The listing builds one solid part. Answer for the finished solid, in the listing's coordinates (mm). Face numbers are marked on the shaded views. A direction names the side the tool comes from. Give positions to 0.01 mm unless a question says otherwise; leave off trailing zeros. Loops run counter-clockwise (first coordinate to the right, second up) from the corner with the lowest first, then second, coordinate; pieces in that order, holes last. Notation, with made-up numbers: M -17.75,75 L 24.25,75 A28 cw 24.25,105 Z; hole C -38.5,-31 d9. An arc over 180 degrees is marked long. Return JSON: item names as keys, results as strings.
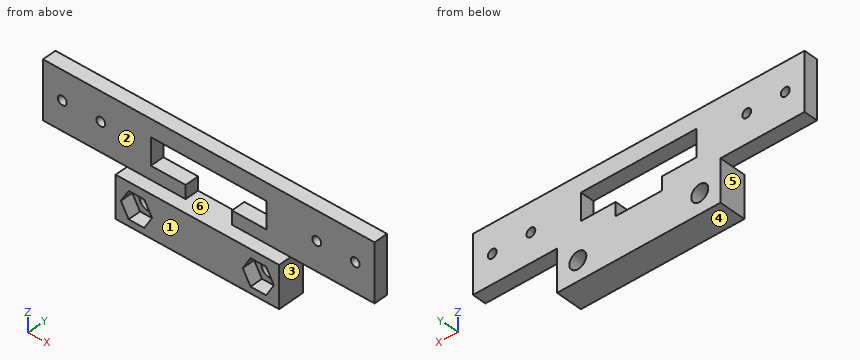
from build123d import *

# Parameters (mm, degrees)
SKETCH1_R           = 1.15
SKETCH1_R_2         = 2.2
BOSS_EXTRUDE2_DEPTH = 3.6
SKETCH2_W           = 42.4
SKETCH2_H           = 10.88
BOSS_EXTRUDE3_DEPTH = 3.3


with BuildPart() as part:
    # Sketch1 → Boss-Extrude2 (new body)
    with BuildSketch(Plane(origin=(0, 0, 0), x_dir=(1, 0, 0), z_dir=(0, 1, 0))):
        Polygon((33, 7.5), (21.2, 7.5), (21.2, 18.38), (-21.2, 18.38), (-21.2, 7.5), (-33, 7.5), (-43, 7.5), (-43, -7.5), (43, -7.5), (43, 7.5), align=None)
        Polygon((-15, -3), (-15, 4), (-6, 4), (-6, 7.5), (0, 7.5), (6, 7.5), (6, 4), (15, 4), (15, -3), align=None, mode=Mode.SUBTRACT)
        with Locations((-38, 0)):
            Circle(SKETCH1_R, mode=Mode.SUBTRACT)
        with Locations((-28, 0)):
            Circle(SKETCH1_R, mode=Mode.SUBTRACT)
        with Locations((28, 0)):
            Circle(SKETCH1_R, mode=Mode.SUBTRACT)
        with Locations((38, 0)):
            Circle(SKETCH1_R, mode=Mode.SUBTRACT)
        with Locations((-15.81, 13.2)):
            Circle(SKETCH1_R_2, mode=Mode.SUBTRACT)
        with Locations((15.81, 13.2)):
            Circle(SKETCH1_R_2, mode=Mode.SUBTRACT)
    extrude(amount=BOSS_EXTRUDE2_DEPTH)

    # Sketch2 → Boss-Extrude3 (add)
    with BuildSketch(Plane.XZ):
        with Locations((0, -12.94)):
            Rectangle(SKETCH2_W, SKETCH2_H)
        Polygon((-11.768548116, -13.2), (-13.789274058, -9.7), (-17.830725942, -9.7), (-19.851451884, -13.2), (-17.830725942, -16.7), (-13.789274058, -16.7), align=None, mode=Mode.SUBTRACT)
        Polygon((19.851451884, -13.2), (17.830725942, -9.7), (13.789274058, -9.7), (11.768548116, -13.2), (13.789274058, -16.7), (17.830725942, -16.7), align=None, mode=Mode.SUBTRACT)
    extrude(amount=BOSS_EXTRUDE3_DEPTH)


solid = part.part
(1) The part is cut by section C-C (y = -2). Determine the outline of the cut face in (x, z), and give its area (3 significant figures).
Values follow:
{"outline": "M -21.2,-18.38 L 21.2,-18.38 L 21.2,-7.5 L -21.2,-7.5 Z; hole M -19.85,-13.2 L -17.83,-16.7 L -13.79,-16.7 L -11.77,-13.2 L -13.79,-9.7 L -17.83,-9.7 Z; hole M 11.77,-13.2 L 13.79,-16.7 L 17.83,-16.7 L 19.85,-13.2 L 17.83,-9.7 L 13.79,-9.7 Z", "area": "376 mm²"}
(2) The part is cut by section A-A (z = -2.5). Determine the outline of the cut face in (x, y), and give its area (3 significant figures).
Values follow:
{"outline": "M -43,0 L -15,0 L -15,3.6 L -43,3.6 Z; M 15,0 L 43,0 L 43,3.6 L 15,3.6 Z", "area": "202 mm²"}
(3) Determine the mould class of the marked faces 4, 5 and 6 for opening direction X: released by +X, released by -X, zero draft, split by the parting line, or undercut.
Values follow:
{"face 4": "zero draft", "face 5": "released by -X", "face 6": "undercut"}
(4) Given pin 1 (2.5 mm diameter, centred on x = 15, y = -1.5, fed in from +Z); pin 2 (12 mm diameter, centred on x = 20, z = 2.5, fed in from -Y); pin 3 (3 mm diameter, centred on x = 37, y = 1, fed in from -Z), each flat-ended and moving along its own axis, determine where each tip first touches the part or whether it passes through.
Values follow:
{"pin 1": "z = -7.5", "pin 2": "y = 0", "pin 3": "z = -7.5"}
(5) Straight lines are drawn through the part: line 1 along X through (y, z) = (1.35, -13.2); line 2 along X through (y, z) = (2.05, 0); line 3 along Z through (x, y) = (38, 1.5). For each, find the intervals that lie inside material, in ascending order.
Values follow:
{"line 1": "-21.2 to -18.01, -13.61 to 13.61, 18.01 to 21.2", "line 2": "-43 to -39.15, -36.85 to -29.15, -26.85 to -15, 15 to 26.85, 29.15 to 36.85, 39.15 to 43", "line 3": "-7.5 to -1.15, 1.15 to 7.5"}
(6) A tool of negligible diameter and unlimited length cuts with its end or side. For the marked faces 1, 2 and 3, from which of +Z, -Z, +X, -X, +Y, -Y can it reach the whole face along a straight path? Write none if from no direction.
Values follow:
{"face 1": "+Z, -Z, +X, -X, -Y", "face 2": "+Z, +X, -X, -Y", "face 3": "-Z, +X, +Y, -Y"}
(7) The part is cut by section B-B (x = -28). Determine the outline of the cut face in (y, z).
Values follow:
{"outline": "M 0,-7.5 L 3.6,-7.5 L 3.6,-1.15 L 0,-1.15 Z; M 0,1.15 L 3.6,1.15 L 3.6,7.5 L 0,7.5 Z"}
(8) The part is cut by section D-D (y = 2.5). Determine the outline of the cut face in (x, z).
Values follow:
{"outline": "M -43,-7.5 L -21.2,-7.5 L -21.2,-18.38 L 21.2,-18.38 L 21.2,-7.5 L 43,-7.5 L 43,7.5 L -43,7.5 Z; hole C -38,0 d2.3; hole C -28,0 d2.3; hole C -15.81,-13.2 d4.4; hole M -15,-4 L -6,-4 L -6,-7.5 L 6,-7.5 L 6,-4 L 15,-4 L 15,3 L -15,3 Z; hole C 15.81,-13.2 d4.4; hole C 28,0 d2.3; hole C 38,0 d2.3"}
